from build123d import *

# Parameters (mm, degrees)
SKETCH1_R           = 3.175
BOSS_EXTRUDE1_DEPTH = 6.35


with BuildPart() as part:
    # Sketch1 → Boss-Extrude1 (new body)
    with BuildSketch(Plane.XY):
        Polygon((12.7, 0), (38.1, 0), (38.1, -6.35), (50.8, -6.35), (50.8, 0), (50.8, 101.6), (0, 101.6), (0, 0), (0, -6.35), (12.7, -6.35), align=None)
        with Locations((12.7, 76.2)):
            Circle(SKETCH1_R, mode=Mode.SUBTRACT)
        with Locations(Location((38.1, 76.2, 0), (0, 0, 180))):
            Circle(SKETCH1_R, mode=Mode.SUBTRACT)
        with Locations((12.7, 38.1)):
            Circle(SKETCH1_R, mode=Mode.SUBTRACT)
        with Locations(Location((38.1, 38.1, 0), (0, 0, 180))):
            Circle(SKETCH1_R, mode=Mode.SUBTRACT)
    extrude(amount=BOSS_EXTRUDE1_DEPTH)


solid = part.part
The model under review builds one solid part; all positions refer to its coordinate system, in mm. A direction names the side the tool comes from. Give positions to 0.01 mm unless a question says otherwise; leave off trailing zeros. Order: outer loops, then holes, each group sorted by start corner. A loop starts at its lowest first (then second) coordinate and runs counter-clockwise, first axis right, second up. Notation, with made-up numbers: M 31.25,33 L 52.25,33 A24 ccw 52.25,71 Z; hole C -39.5,88.25 d5. An arc over 180 degrees is marked long. Use one line per item in the form item = value. Start each with the question number.
Item 1: We need section C-C on x = 26.5. Give the boundary of the cut face in (y, z), plus the area to 3 significant figures.
Item 2: We need section B-B on y = 76.2. Give the boundary of the cut face in (x, z) (3 decimals).
Item 3: For faces 5 (the flat face through (38.1, -3, 3)), 6 (the flat face through (26, 101.6, 3)), list the 3-axis set-ups (+Z, -Z, +X, -X, +Y, -Y) from which the entire face can be reached by the end or side of a thin tool; tool diameter is ignored.
Item 4: Insertion check: pin 1 Ø1.5 at (x, y) = (39, 42) entering from -Z; pin 2 Ø3 at (x, z) = (24, 3.5) entering from -Y. Each pin has a flat end and moves straight along its axis. Give the tip position at first contact, or say it passes through.
Item 5: We need section A-A on z = 1.25. Give the boundary of the cut face in (x, y) (3 decimals).
Item 6: The part is to be moulded in two halves that separate along X. For faces 1 (the flat face through (25, 48, 6.35)), 2 (the flat face through (25, 0, 3)), 3 (the cylindrical face through (10.18, 36.17, 3.13)), 4 (the flat face through (0, 48, 3)), say which applies: pulls with the +X half, pulls with the -X half, needs draft (parallel to the pull), parting line crosses it, or undercut.
Item 7: To check wall thickness, follow line 1 along Y through (x, z) = (38, 5.75); line 2 along Y through (x, z) = (12, 4.5); line 3 along Y through (x, z) = (22, 1.25). State the ranges of each line that lie inside material, in increasing order. Write a range as from..to.
Completed:
q1.outline = M 0,0 L 101.6,0 L 101.6,6.35 L 0,6.35 Z
q1.area = 645 mm²
q2.outline = M 0,0 L 9.525,0 L 9.525,6.35 L 0,6.35 Z; M 15.875,0 L 34.925,0 L 34.925,6.35 L 15.875,6.35 Z; M 41.275,0 L 50.8,0 L 50.8,6.35 L 41.275,6.35 Z
q3.face_5 = +Z, -Z, -Y
q3.face_6 = +Z, -Z, +X, -X, +Y
q4.pin_1 = 0
q4.pin_2 = 0
q5.outline = M 0,-6.35 L 12.7,-6.35 L 12.7,0 L 38.1,0 L 38.1,-6.35 L 50.8,-6.35 L 50.8,101.6 L 0,101.6 Z; hole C 12.7,38.1 d6.35; hole C 12.7,76.2 d6.35; hole C 38.1,38.1 d6.35; hole C 38.1,76.2 d6.35
q6.face_1 = needs draft
q6.face_2 = undercut
q6.face_3 = undercut
q6.face_4 = pulls with the -X half
q7.line_1 = 0..34.93, 41.27..73.03, 79.37..101.6
q7.line_2 = -6.35..35, 41.2..73.1, 79.3..101.6
q7.line_3 = 0..101.6
